Geometry: see drawing. Coordinates: mm, zero at the bounding-box minimum. A direction names the side the tool comes from. Coordinates: 2 decimals unless noted, no trailing zeros. Order: outer loops, then holes, each group sorted by start corner. A loop starts at its lowest first (then second) coordinate and runs counter-clockwise, first axis right, second up. Notation, with made-up numbers: (19, 30.5) -> (68, 30.5) arc R21 cw to (68, 46.5) -> close; hole circle Ø3 at (62.5, -38.5). An arc over 180 degrees is marked (long way). Use one line per item in the form item = value.
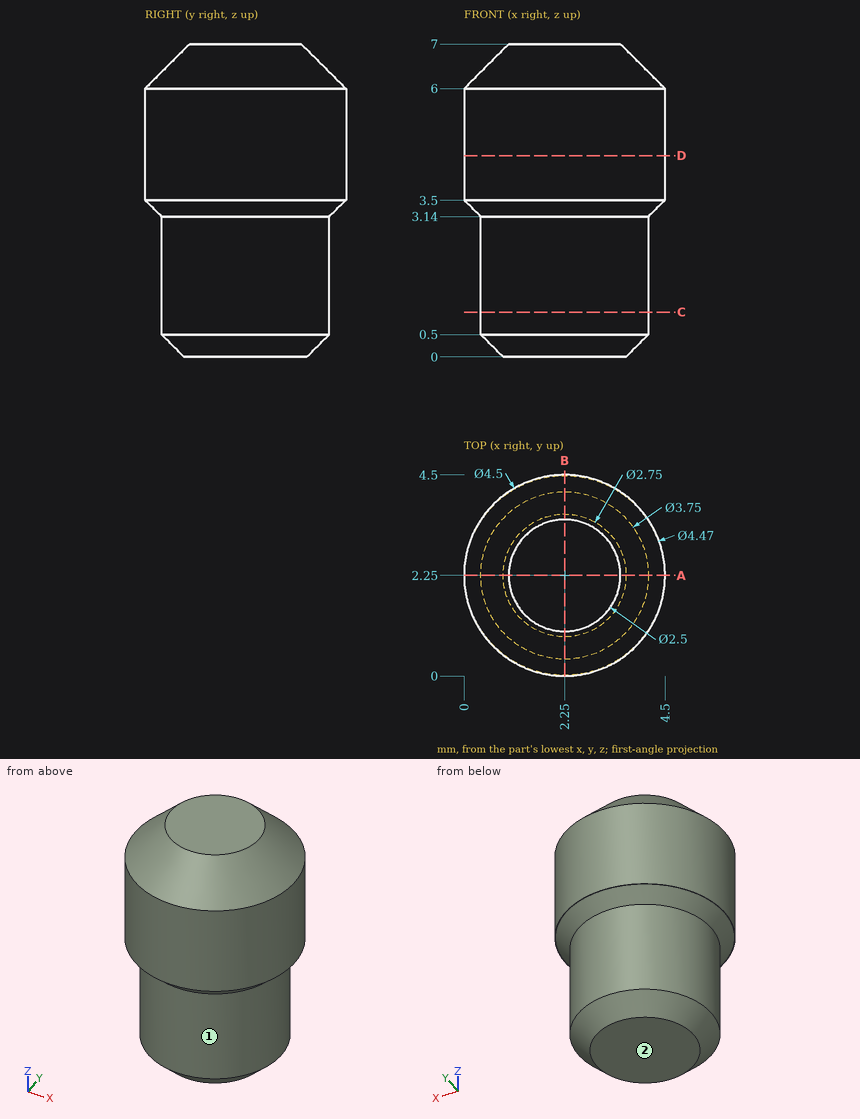
1) Material intervals for probe 1 along X at (y, z) = (2.3, 1.75); probe 2 along Z at (x, y) = (0.85, 2.25) (3 decimals); probe 3 along Y at (x, z) = (1.95, 5.25), sorted ascending. Write a range as from..to.
Results found:
probe_1 = 0.38..4.12
probe_2 = 0.025..6.85
probe_3 = 0.02..4.48
2) Section A-A, the plane y = 2.25. Output: boundary loops of the cut face in (x, z) (3 decimals).
Results found:
outline = (0, 3.5) -> (0.015, 3.5) -> (0.375, 3.14) -> (0.375, 0.5) -> (0.875, 0) -> (3.625, 0) -> (4.125, 0.5) -> (4.125, 3.14) -> (4.485, 3.5) -> (4.5, 3.5) -> (4.5, 6) -> (3.5, 7) -> (1, 7) -> (0, 6) -> close
3) Section D-D, the plane z = 4.5. Output: boundary loops of the cut face in (x, y).
Results found:
outline = circle Ø4.5 at (2.25, 2.25)
4) Section C-C, the plane z = 1. Output: boundary loops of the cut face in (x, y) (3 decimals), and give its area (3 significant figures).
Results found:
outline = circle Ø3.75 at (2.25, 2.25)
area = 11.0 mm2
5) Contact query for a flat-ended pin moving along its axis: P1, Ø1, axis at x = 3.5, z = 4, coming from the -Y side. Output: stop coordinate, or through.
Results found:
P1 = 0.13
6) Access query for the marked faces 1 and 2. Directions: +Z, -Z, +X, -X, +Y, -Y. A direction counts if a zero-diameter tool reaches every point of the face in a straight line with its end or side. Return the directions, or none.
Results found:
face_1 = -Z
face_2 = -Z, +X, -X, +Y, -Y
